from build123d import *

# Parameters (mm, degrees)
SKETCH3_R           = 48.7045
BOSS_EXTRUDE1_DEPTH = 76.2
SKETCH4_R           = 12.7
SKETCH5_R           = 48.7045
SKETCH5_R_2         = 12.7
BOSS_EXTRUDE2_DEPTH = 25.4
SKETCH6_R           = 3.429
CUT_EXTRUDE1_DEPTH  = 355.6


with BuildPart() as part:
    # Sketch2 → Revolve1 (revolve)
    with BuildSketch(Plane.XY):
        with BuildLine():
            Line((-1e-09, 0), (508, 0))
            Line((508, 0), (508, 51.1048))
            add(Edge.make_bspline(
                [(-1e-09, 0), (0.711812873, 0.144680974), (2.158225426, 0.437865374), (5.390910998, 1.091290389), (8.4055347, 1.694324361), (12.023782781, 2.415194505), (15.32985135, 3.067757265), (18.81147443, 3.751148051), (22.194233026, 4.409589314), (25.653426609, 5.078524787), (29.101387687, 5.740045977), (33.459511631, 6.570152036), (38.703794572, 7.558802799), (44.830842505, 8.699211823), (51.833102117, 9.982239097), (58.840911875, 11.246114682), (65.851059887, 12.490186989), (72.865349703, 13.714824009), (79.882611918, 14.919789625), (86.903462237, 16.105210706), (93.927446457, 17.270996817), (100.95474067, 18.417185788), (109.742774093, 19.825383246), (120.294674252, 21.475961868), (146.693369586, 25.479624229), (189.013226456, 31.334973644), (234.983464044, 36.738785793), (281.060072425, 41.114345359), (312.999037596, 43.668169814), (330.752870377, 44.954816779), (344.961441701, 45.904815612), (359.175131847, 46.775466104), (371.61611191, 47.467831729), (382.282525687, 48.011662883), (391.172664946, 48.431765176), (398.285951755, 48.747990192), (405.399564609, 49.044355925), (412.514881745, 49.320860063), (421.408249235, 49.641660547), (430.30556766, 49.929351449), (439.199267742, 50.183928153), (448.100682593, 50.405386823), (455.212245734, 50.562681557), (462.343887521, 50.700102863), (468.551333113, 50.80295632), (473.924175337, 50.878694291), (479.17080941, 50.944021455), (484.543653599, 50.999186043), (490.444224468, 51.049296261), (496.881841793, 51.082598465), (501.585135763, 51.099249612), (505.808857653, 51.104007087), (507.273632283, 51.1048), (508, 51.1048)],
                knots=[0.083030368, 0.083030368, 0.083030368, 0.083030368, 0.083030368, 0.088711546, 0.094392725, 0.100073903, 0.105755081, 0.111436259, 0.117117438, 0.122798616, 0.128479794, 0.134286138, 0.140092482, 0.151705171, 0.163317859, 0.174930547, 0.186543236, 0.198155925, 0.209768614, 0.221381304, 0.232993993, 0.244606682, 0.256219371, 0.26783206, 0.291057438, 0.314282816, 0.430409703, 0.546536592, 0.592987348, 0.616212726, 0.639438104, 0.662663482, 0.685888859, 0.709114237, 0.720726926, 0.732339615, 0.743952304, 0.755564993, 0.767177681, 0.77879037, 0.802015748, 0.813628437, 0.825241126, 0.836853815, 0.848466503, 0.860079192, 0.865885537, 0.871691881, 0.883054237, 0.894416592, 0.905778948, 0.911460125, 0.917141303, 0.917141303, 0.917141303, 0.917141303, 0.917141303], degree=4))
        make_face()
    revolve(axis=Axis((-1e-09, 0, 0), (1, 0, 0)))

    # Sketch3 → Boss-Extrude1 (add)
    with BuildSketch(Plane(origin=(508, 0, 0), x_dir=(0, 0, -1), z_dir=(1, 0, 0))):
        with Locations(Location((0, 0, 0), (0, 0, 180))):
            Circle(SKETCH3_R)
    extrude(amount=BOSS_EXTRUDE1_DEPTH)

    # Sketch4 → Cut-Revolve1 (revolve, cut)
    with BuildSketch(Plane(origin=(584.2, 0, 0), x_dir=(0, 0, -1), z_dir=(1, 0, 0)), mode=Mode.PRIVATE) as cut_revolve1_sk:
        with Locations((-25.4, 0)):
            Circle(SKETCH4_R)
    revolve(cut_revolve1_sk.sketch.rotate(Axis((584.2, 48.7045, 0), (0, -1, 0)), 90), axis=Axis((584.2, 48.7045, 0), (0, -1, 0)), mode=Mode.SUBTRACT)

    # Sketch5 → Boss-Extrude2 (add)
    with BuildSketch(Plane(origin=(584.2, 0, 0), x_dir=(0, 0, -1), z_dir=(1, 0, 0))):
        with Locations(Location((0, 0, 0), (0, 0, 180))):
            Circle(SKETCH5_R)
        with Locations(Location((-25.4, 0, 0), (0, 0, 180))):
            Circle(SKETCH5_R_2, mode=Mode.SUBTRACT)
        with Locations((25.4, 0)):
            Circle(SKETCH5_R_2, mode=Mode.SUBTRACT)
    extrude(amount=BOSS_EXTRUDE2_DEPTH)

    # Sketch6 → Cut-Extrude1 (cut)
    with BuildSketch(Plane(origin=(609.6, 0, 0), x_dir=(0, 0, -1), z_dir=(1, 0, 0))):
        with Locations((0, 25.4)):
            Circle(SKETCH6_R)
        with Locations((0, -25.4)):
            Circle(SKETCH6_R)
    extrude(amount=-CUT_EXTRUDE1_DEPTH, mode=Mode.SUBTRACT)


solid = part.part
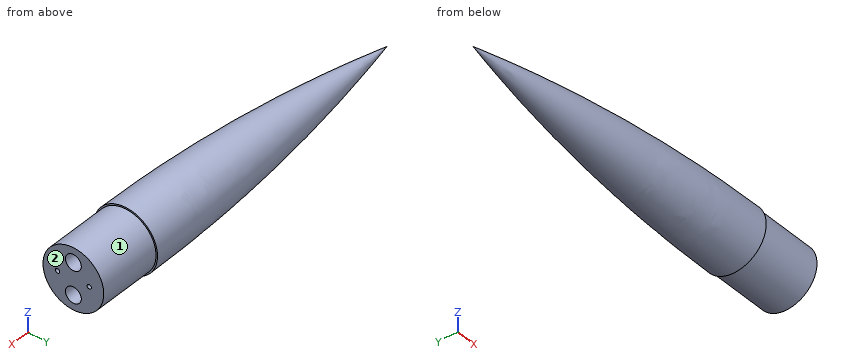
Input: part model. Units: mm. Frame: model coordinates. Face numbers are marked on the shaded views. A direction names the side the tool comes from. Coordinates: 2 decimals unless noted, no trailing zeros.
(1) Section A-A on x = 434.5. Count the separate pieces of the cut face and the enclosed holes in it, then the cut area to 3 significant figures.
(2) First-contact query: pin 1 Ø4 at (y, z) = (39.5, 37) entering from +X (3 decimals); pin 2 Ø4 at (x, z) = (343, -6) entering from +Y; pin 3 Ø5 at (x, y) = (200, -12.5) entering from -Z; pin 4 Ø8 at (x, z) = (374, 14) entering from +Y. Flat tips, straight axial feed; report the tip coordinate or a pass-through.
(3) Set-up query: the marked faces 1 and 2. Return all of +Z, -Z, +X, -X, +Y, -Y with unobstructed straight access to the full face (end or side cutting, diameter ignored); none if empty.
(4) Material intervals for probe 1 along Y at (x, z) = (423, 0); probe 2 along Y at (x, z) = (364, 0); probe 3 along Y at (x, z) = (598.5, 25.4), sorted ascending.
Data:
1. separate pieces: 1
1. enclosed holes: 2
1. area: 7,790 mm2
2. pin 1: passes through
2. pin 2: stops at y = 45.63
2. pin 3: stops at z = -30.92
2. pin 4: stops at y = 46.55
3. face 1: +X
3. face 2: +Z, -Z, +X, +Y, -Y
4. probe 1: y = -49.69 to -28.83, -21.97 to 21.97, 28.83 to 49.69
4. probe 2: y = -47.04 to -28.83, -21.97 to 21.97, 28.83 to 47.04
4. probe 3: y = -41.56 to -12.7, 12.7 to 41.56
